Check sheet for the modelled part. Datum: model origin and axes. Units: mm. A direction names the side the tool comes from. Round coordinates to 2 decimals unless told otherwise and drop trailing zeros. Order: outer loops, then holes, each group sorted by start corner. A loop starts at its lowest first (then second) coordinate and runs counter-clockwise, first axis right, second up. Notation, with made-up numbers: (-25, 7.5) -> (15, 7.5) arc R13 ccw to (15, 23.5) -> close; hole circle Ø6 at (76.25, -28.5). An arc over 180 degrees is marked (long way). Use CSV: the item, a comma, the result in double quotes.
```python
from build123d import *

# Parameters (mm, degrees)
F0_W     = 152.4
F0_H     = 50.8
F1_DEPTH = 76.2
F3_DEPTH = 76.201
F5_DEPTH = 76.201
F7_DEPTH = 152.401


with BuildPart() as f1:
    # F0 (on Front) → F1 (new body)
    with BuildSketch(Plane.XZ):
        with Locations((-45.980399, 37.487842)):
            Rectangle(F0_W, F0_H)
    extrude(amount=F1_DEPTH)

    # F2 (on face) → F3 (cut, through all)
    with BuildSketch(Plane.XZ.offset(76.2)):
        Polygon((-71.380399, 62.887842), (-96.780399, 62.887842), (-96.780399, 50.187842), (-109.480399, 50.187842), (-109.480399, 37.487842), (-58.680399, 37.487842), (-58.680399, 50.187842), (-71.380399, 50.187842), align=None)
    extrude(amount=-F3_DEPTH, mode=Mode.SUBTRACT)

    # F4 (on face) → F5 (cut, through all)
    with BuildSketch(Plane.XZ.offset(76.2)):
        Polygon((30.219601, 62.887842), (-45.980399, 62.887842), (-39.970737, 52.092843), (30.219601, 52.092843), align=None)
    extrude(amount=-F5_DEPTH, mode=Mode.SUBTRACT)

    # F6 (on face) → F7 (cut, through all)
    with BuildSketch(Plane.YZ.offset(30.219601)):
        Polygon((-61.302628, 20.722013), (-50.8, 12.087842), (-25.4, 12.087842), (-10.502628, 20.722013), align=None)
    extrude(amount=-F7_DEPTH, mode=Mode.SUBTRACT)


solid = f1.part
```
Q1. Sectioned sample at A-A, the plane x = -77.5. Enter the section's corners in (y, z), then the cut area to 3 significant figures.
Result sheet:
outline,"(-76.2, 12.09) -> (-50.8, 12.09) -> (-61.3, 20.72) -> (-10.5, 20.72) -> (-25.4, 12.09) -> (0, 12.09) -> (0, 37.49) -> (-76.2, 37.49) -> close"
area,"1,610 mm^2"
Q2. Sectioned sample at D-D, the plane x = -33. Enter the section's corners in (y, z).
Result sheet:
outline,"(-76.2, 12.09) -> (-50.8, 12.09) -> (-61.3, 20.72) -> (-10.5, 20.72) -> (-25.4, 12.09) -> (0, 12.09) -> (0, 52.09) -> (-76.2, 52.09) -> close"
Q3. Go/stop test with flat-tipped pins: pin 1 (6 mm diameter, centred on x = -40, y = -30, fed in from -Z); pin 2 (4 mm diameter, centred on y = -44, z = 57, fed in from +X); pin 3 (4 mm diameter, centred on y = -41.5, z = 55, fed in from +X). Record where each tip stops, or that it passes through.
Result sheet:
pin 1,"stops at z = 20.72"
pin 2,"stops at x = -41.59"
pin 3,"stops at x = -40.48"
Q4. Sectioned sample at B-B, the plane y = -6.5. Enter the section's corners in (x, z).
Result sheet:
outline,"(-122.18, 12.09) -> (30.22, 12.09) -> (30.22, 52.09) -> (-39.97, 52.09) -> (-45.98, 62.89) -> (-71.38, 62.89) -> (-71.38, 50.19) -> (-58.68, 50.19) -> (-58.68, 37.49) -> (-109.48, 37.49) -> (-109.48, 50.19) -> (-96.78, 50.19) -> (-96.78, 62.89) -> (-122.18, 62.89) -> close"
Q5. Scan lines: L1, parallel to Z at x = -64, y = -63; L2, parallel to Z at x = -60.5, y = -42.5; L3, parallel to Z at x = -14.5, y = -32. Record each from-to range of solid material in increasing order.
Result sheet:
L1,"z = 12.09 to 37.49, 50.19 to 62.89"
L2,"z = 20.72 to 37.49, 50.19 to 62.89"
L3,"z = 20.72 to 52.09"
Q6. Sectioned sample at C-C, the plane z = 17.5. Enter the section's corners in (x, y).
Result sheet:
outline,"(-122.18, -76.2) -> (30.22, -76.2) -> (30.22, -57.38) -> (-122.18, -57.38) -> close; (-122.18, -16.06) -> (30.22, -16.06) -> (30.22, 0) -> (-122.18, 0) -> close"
Q7. Access from +Z, -Z, +X, -X, +Y, -Y to the whole of each face (thin tool, end or side, straight path). Record for faces 1 (the face through (-71.38, -39, 56)), 2 (the face through (-5, -39, 52.093)), 3 (the face through (-45, -36, 20.722)), 4 (the face through (-65, -39, 50.188)).
Result sheet:
face 1,"+Z, +Y, -Y"
face 2,"+Z, +X, +Y, -Y"
face 3,"+X, -X"
face 4,"+Y, -Y"
Q8. Mould release check, pull along X, two halves, no side actions. Record for faces 5 (the face through (-122.18, -38, 37)), 6 (the face through (-47, -63, 12.088)), 7 (the face through (-43.02, -38.63, 57.57)), 8 (the face through (-58.68, -39, 44)): pulls with the +X half, pulls with the -X half, needs draft (parallel to the pull), parting line crosses it, or undercut.
Result sheet:
face 5,"pulls with the -X half"
face 6,"needs draft"
face 7,"pulls with the +X half"
face 8,"undercut"
